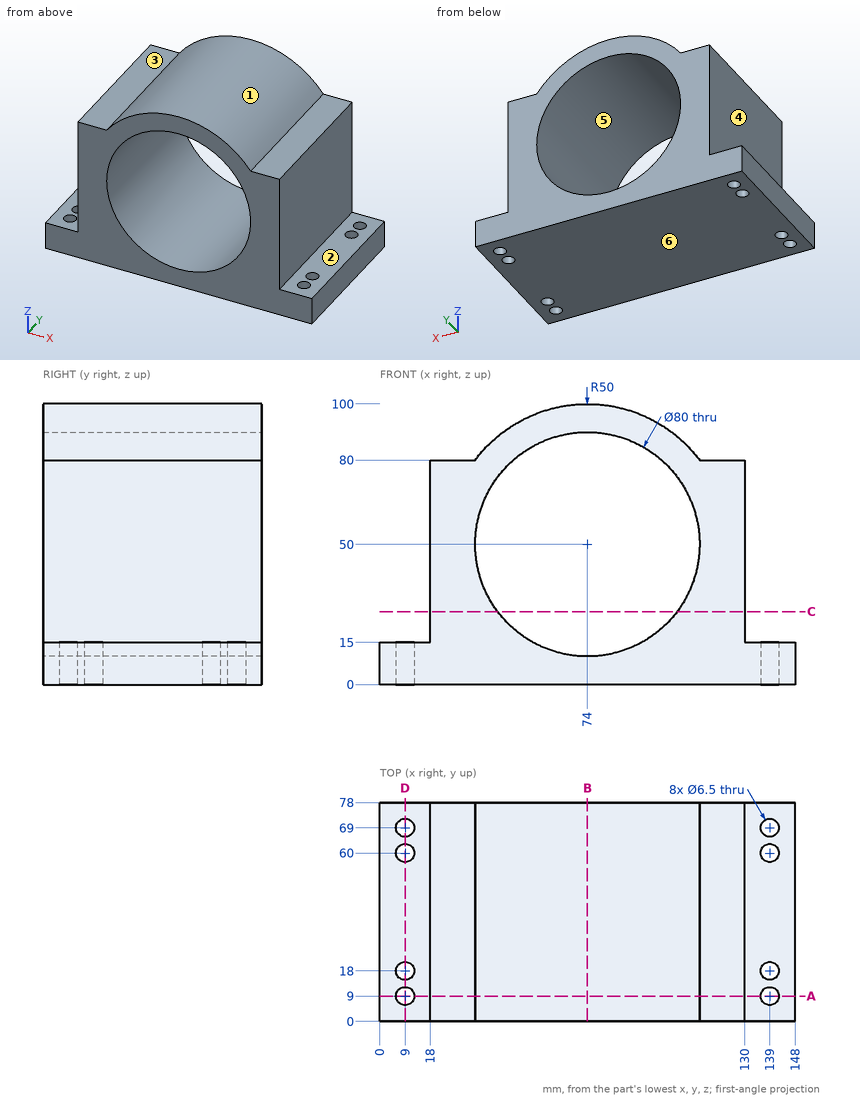
Here's the drawing with two shaded views (mm, measured from the low corner). I have some questions. A direction names the side the tool comes from. Coordinates: 2 decimals unless noted, no trailing zeros. Order: outer loops, then holes, each group sorted by start corner. A loop starts at its lowest first (then second) coordinate and runs counter-clockwise, first axis right, second up.
Item 1: I need wall thicknesses on line 1 (Y direction, x = 139, z = 8); line 2 (X direction, y = 37, z = 50); line 3 (Z direction, x = 73.5, y = 21). Which ranges of each line are inside material? Lowest first, please.
Result sheet:
line 1: y = 0 to 5.75, 12.25 to 14.75, 21.25 to 56.75, 63.25 to 65.75, 72.25 to 78
line 2: x = 18 to 34, 114 to 130
line 3: z = 0 to 10, 90 to 100
Item 2: For P1, Ø8.5, axis at x = 139, y = 69, coming from the -Z side; P2, Ø8.5, axis at x = 9, y = 69, coming from the +Z side; P3, Ø4, axis at x = 27, y = 8, coming from the +Z side; P4, Ø3, axis at x = 55.5, y = 24.5, coming from the +Z side, each with a flat end and sliding along its axis, tell me the tip position at first contact or that it passes through.
Result sheet:
P1: stops at z = 0
P2: stops at z = 15
P3: stops at z = 80
P4: stops at z = 97.02
Item 3: For the marked faces 1, 2 and 3, which set-ups out of +Z, -Z, +X, -X, +Y, -Y let a thin tool reach every point of the face, with its end or its side?
Result sheet:
face 1: +Z, +Y, -Y
face 2: +Z, +X, +Y, -Y
face 3: +Z, -X, +Y, -Y
Item 4: If we section it at D-D on x = 9: List the corners of the cut face in (y, z) for me.
Result sheet:
outline: (0, 0) - (5.75, 0) - (5.75, 15) - (0, 15) - close; (12.25, 0) - (14.75, 0) - (14.75, 15) - (12.25, 15) - close; (21.25, 0) - (56.75, 0) - (56.75, 15) - (21.25, 15) - close; (63.25, 0) - (65.75, 0) - (65.75, 15) - (63.25, 15) - close; (72.25, 0) - (78, 0) - (78, 15) - (72.25, 15) - close
Item 5: If we section it at A-A on y = 9: List the corners of the cut face in (x, z) for me, plus the area to 3 significant figures.
Result sheet:
outline: (0, 0) - (5.75, 0) - (5.75, 15) - (0, 15) - close; (12.25, 0) - (135.75, 0) - (135.75, 15) - (130, 15) - (130, 80) - (114, 80) arc R50 ccw to (34, 80) - (18, 80) - (18, 15) - (12.25, 15) - close; (142.25, 0) - (148, 0) - (148, 15) - (142.25, 15) - close; hole circle Ø80 at (74, 50)
area: 5,400 mm2
Item 6: If we section it at C-C on z = 26: List the corners of the cut face in (x, y) for me.
Result sheet:
outline: (18, 0) - (42, 0) - (42, 78) - (18, 78) - close; (106, 0) - (130, 0) - (130, 78) - (106, 78) - close
Item 7: If we mould it in two halves opening along Z, with no side actions, what happens to the marked faces 4, 5 and 6? For each: +Z half, -Z half, draft (parallel to the pull), parting line (faces both ways), or undercut.
Result sheet:
face 4: draft
face 5: undercut
face 6: -Z half
Item 8: If we section it at B-B on x = 74: List the corners of the cut face in (y, z) for me.
Result sheet:
outline: (0, 0) - (78, 0) - (78, 10) - (0, 10) - close; (0, 90) - (78, 90) - (78, 100) - (0, 100) - close
